The model under review builds one solid part; all positions refer to its coordinate system, in mm. A direction names the side the tool comes from. Coordinates: 2 decimals unless noted, no trailing zeros. Loops run counter-clockwise (first coordinate to the right, second up) from the corner with the lowest first, then second, coordinate; pieces in that order, holes last. Notation, with made-up numbers: M 64.25,83.25 L 107.25,83.25 A22 ccw 107.25,110.25 Z; hole C 49.5,-11 d8. An arc over 180 degrees is marked long. Return JSON: item names as keys, results as strings.
```python
from build123d import *

# Parameters (mm, degrees)
SKETCH2_R           = 5
BOSS_EXTRUDE1_DEPTH = 7
BOSS_EXTRUDE2_DEPTH = 12.5
BOSS_EXTRUDE3_DEPTH = 0.2
SKETCH5_R           = 2
BOSS_EXTRUDE4_DEPTH = 1


with BuildPart() as part:
    # Sketch2 → Boss-Extrude1 (new body)
    with BuildSketch(Plane(origin=(0, 0, 0), x_dir=(1, 0, 0), z_dir=(0, 1, 0))):
        with Locations(Location((0, 0, 0), (0, 0, 270))):
            Circle(SKETCH2_R)
    extrude(amount=BOSS_EXTRUDE1_DEPTH)

    # Sketch3 → Boss-Extrude2 (add)
    with BuildSketch(Plane(origin=(0, 7, 0), x_dir=(1, 0, 0), z_dir=(0, 1, 0))):
        with BuildLine():
            Line((-3.975, 2.99165506), (-3.975, -2.99165506))
            ThreePointArc((-3.975, -2.99165506), (0, -4.975), (3.975, -2.99165506))
            Line((3.975, -2.99165506), (3.975, 2.99165506))
            ThreePointArc((3.975, 2.99165506), (0, 4.975), (-3.975, 2.99165506))
        make_face()
    extrude(amount=BOSS_EXTRUDE2_DEPTH)

    # Sketch4 → Boss-Extrude3 (add)
    with BuildSketch(Plane(origin=(0, 19.5, 0), x_dir=(1, 0, 0), z_dir=(0, 1, 0))):
        with BuildLine():
            Line((-3.2, 3.5), (-2.1, 3.5))
            ThreePointArc((-2.1, 3.5), (-1.569669914, 3.280330086), (-1.35, 2.75))
            Line((-1.35, 2.75), (-1.35, -5))
            Line((-1.35, -5), (-3.95, -5))
            Line((-3.95, -5), (-3.95, 2.75))
            ThreePointArc((-3.95, 2.75), (-3.730330086, 3.280330086), (-3.2, 3.5))
        make_face()
        with BuildLine():
            Line((3.95, -5), (1.35, -5))
            Line((1.35, -5), (1.35, 2.75))
            ThreePointArc((1.35, 2.75), (1.569669914, 3.280330086), (2.1, 3.5))
            Line((2.1, 3.5), (3.2, 3.5))
            ThreePointArc((3.2, 3.5), (3.730330086, 3.280330086), (3.95, 2.75))
            Line((3.95, 2.75), (3.95, -5))
        make_face()
    extrude(amount=BOSS_EXTRUDE3_DEPTH)

    # Sketch5 → Boss-Extrude4 (add)
    with BuildSketch(Plane(origin=(0, 19.5, 0), x_dir=(1, 0, 0), z_dir=(0, 1, 0))):
        with Locations(Location((0, 0, 0), (0, 0, 47.545849796))):
            Circle(SKETCH5_R)
    extrude(amount=BOSS_EXTRUDE4_DEPTH)


solid = part.part
```
1. The part is to be moulded in two halves that separate along Y. For faces 5 (the face through (-4.88, 3.45, -1.08)), 6 (the face through (-0.064, 13.162, 4.975)), 7 (the face through (0, 20.5, 0)), 8 (the face through (0, 0, 0)), say which applies: released by +Y, released by -Y, zero draft, split by the parting line, or undercut.
Check values:
{"face 5": "zero draft", "face 6": "undercut", "face 7": "released by +Y", "face 8": "released by -Y"}
2. Machinability: for faces 1 (the face through (0, 19.5, 3)), 2 (the face through (0, 19.5, -4)), 3 (the face through (-3.975, 13, 0)), 4 (the face through (3.975, 13, 0)), which of the approach directions +Z, -Z, +X, -X, +Y, -Y give a long, thin tool a straight path to every point of the face, cutting with its end or side? Answer none if there is none.
Check values:
{"face 1": "+Z, +Y", "face 2": "-Z, +Y", "face 3": "+Z, -Z, -X, +Y", "face 4": "+Z, -Z, +X, +Y"}
3. Insertion check: pin 1 Ø2 at (x, z) = (-2, 2.5) entering from +Y; pin 2 Ø1 at (y, z) = (14, 0) entering from +X (3 decimals); pin 3 Ø6 at (y, z) = (4, -3.5) entering from -X. Each pin has a flat end and moves straight along its axis. Give the tip position at first contact, or say it passes through.
Check values:
{"pin 1": "y = 19.7", "pin 2": "x = 3.975", "pin 3": "x = -4.97"}
4. Add section A-A on z = 0. Give the boundary of the cut face in (x, y) (3 decimals).
Check values:
{"outline": "M -5,0 L 5,0 L 5,7 L 3.975,7 L 3.975,19.5 L 3.95,19.5 L 3.95,19.7 L 2,19.7 L 2,20.5 L -2,20.5 L -2,19.7 L -3.95,19.7 L -3.95,19.5 L -3.975,19.5 L -3.975,7 L -5,7 Z"}
5. To check wall thickness, follow line 1 (X direction, y = 17, z = 0.75) (3 decimals); line 2 (Y direction, x = -3.5, z = -0.5); line 3 (Y direction, x = 0.5, z = 2.25). State the ranges of each line that lie inside material, in increasing order.
Check values:
{"line 1": "-3.975 to 3.975", "line 2": "0 to 19.7", "line 3": "0 to 19.5"}
6. Add section B-B on x = 0. Give the boundary of the cut face in (y, z) (3 decimals), plus the area to 3 significant figures.
Check values:
{"outline": "M 0,-5 L 7,-5 L 7,-4.975 L 19.5,-4.975 L 19.5,-2 L 20.5,-2 L 20.5,2 L 19.5,2 L 19.5,4.975 L 7,4.975 L 7,5 L 0,5 Z", "area": "198 mm²"}
